Build history of the part. All positions in model axes, mm. Face numbers are marked on the shaded views. A direction names the side the tool comes from. Round coordinates to 2 decimals unless told otherwise and drop trailing zeros. Loops run counter-clockwise (first coordinate to the right, second up) from the corner with the lowest first, then second, coordinate; pieces in that order, holes last. Notation, with made-up numbers: (-30, 81.25) -> (-20, 81.25) arc R18 cw to (-20, 109.25) -> close; hole circle Ø9 at (0, 74). An arc over 180 degrees is marked (long way). Put each result on its own line as item: value. Start each with the question number.
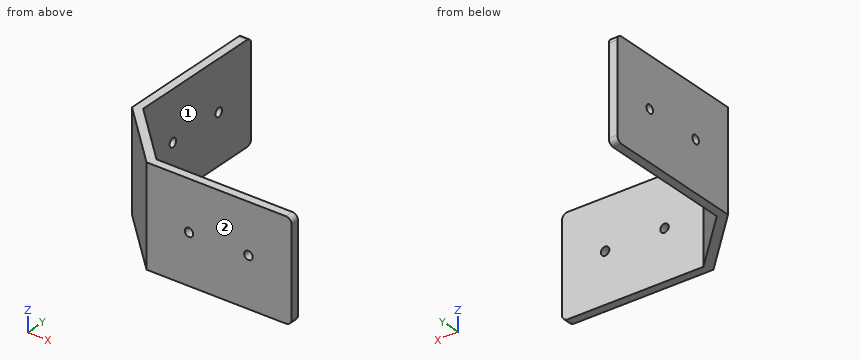
```python
from build123d import *

# Parameters (mm, degrees)
EXTRU_MINCE1_DEPTH      = 35
CONG_3_R                = 2
CONG_4_R                = 2
CONG_5_R                = 2
CONG_6_R                = 2
ESQUISSE2_R             = 1.5
ENL_V_MAT_EXTRU_1_DEPTH = 10
ESQUISSE3_R             = 1.5
ENL_V_MAT_EXTRU_2_DEPTH = 10


with BuildPart() as part:
    # Esquisse1 → Extru.-Mince1 (new body)
    with BuildSketch(Plane.XY):
        Polygon((70, -20), (20, -20), (0, 0), (0, 50), (-3, 50), (-3, -1.242640687), (18.757359313, -23), (70, -23), align=None)
    extrude(amount=EXTRU_MINCE1_DEPTH)

    # Congé3
    cong_3_edges = [part.edges().sort_by_distance(p)[0] for p in [
        (-1.5, 50, 35),
    ]]
    fillet(cong_3_edges, radius=CONG_3_R)

    # Congé4
    cong_4_edges = [part.edges().sort_by_distance(p)[0] for p in [
        (-1.5, 50, 0),
    ]]
    fillet(cong_4_edges, radius=CONG_4_R)

    # Congé5
    cong_5_edges = [part.edges().sort_by_distance(p)[0] for p in [
        (70, -21.5, 35),
    ]]
    fillet(cong_5_edges, radius=CONG_5_R)

    # Congé6
    cong_6_edges = [part.edges().sort_by_distance(p)[0] for p in [
        (70, -21.5, 0),
    ]]
    fillet(cong_6_edges, radius=CONG_6_R)

    # Esquisse2 → Enlèv. mat.-Extru.1 (cut)
    with BuildSketch(Plane.XZ.offset(23)):
        with Locations(Location((33.757359313, 17.5, 0), (0, 0, 270))):
            Circle(ESQUISSE2_R)
        with Locations(Location((54.757359313, 17.5, 0), (0, 0, 270))):
            Circle(ESQUISSE2_R)
    extrude(amount=-ENL_V_MAT_EXTRU_1_DEPTH, mode=Mode.SUBTRACT)

    # Esquisse3 → Enlèv. mat.-Extru.2 (cut)
    with BuildSketch(Plane.ZY.offset(3)):
        with Locations((17.5, 35)):
            Circle(ESQUISSE3_R)
        with Locations((17.5, 13.757359313)):
            Circle(ESQUISSE3_R)
    extrude(amount=-ENL_V_MAT_EXTRU_2_DEPTH, mode=Mode.SUBTRACT)


solid = part.part
```
Item 1: Cut at A-A on z = 17.5. Write the cut outline in (x, y), then the cut area to 3 significant figures.
Item 2: Wall check: line 1 (Y direction, x = -1.6, z = 17.5); line 2 (X direction, y = -21.45, z = 17.5); line 3 (Y direction, x = -1.3, z = 17.5). Give the ranges that are in metal, low to high. Write a range as from..to.
Item 3: Drop flat-ended pins along their axis: pin 1 (12 mm diameter, centred on x = 9.5, z = 8.5, fed in from -Y); pin 2 (12 mm diameter, centred on y = 12.5, z = 25.5, fed in from +X); pin 3 (6 mm diameter, centred on y = -13, z = 20, fed in from +X). Give the stop position or say it passes through.
Item 4: Cut at B-B on y = 35. Write the cut outline in (x, z), then the cut area to 3 significant figures.
Item 5: Cut at C-C on z = 9.5. Write the cut outline in (x, y).
Item 6: 3-axis set-ups, long thin cutter, end or side, ignore diameter. For the marked faces 1 and 2: which of +Z, -Z, +X, -X, +Y, -Y reach the whole face in a straight line?
Item 7: Cut at D-D on y = 24. Write the cut outline in (x, z).
Ans:
1. outline: (-3, -1.24) -> (18.76, -23) -> (32.26, -23) -> (32.26, -20) -> (20, -20) -> (0, 0) -> (0, 12.26) -> (-3, 12.26) -> close; (-3, 15.26) -> (0, 15.26) -> (0, 33.5) -> (-3, 33.5) -> close; (-3, 36.5) -> (0, 36.5) -> (0, 50) -> (-3, 50) -> close; (35.26, -23) -> (53.26, -23) -> (53.26, -20) -> (35.26, -20) -> close; (56.26, -23) -> (70, -23) -> (70, -20) -> (56.26, -20) -> close
1. area: 356 mm2
2. line 1: y = -2.64..12.26, 15.26..33.5, 36.5..50
2. line 2: x = 17.21..32.26, 35.26..53.26, 56.26..70
2. line 3: y = -2.94..12.26, 15.26..33.5, 36.5..50
3. pin 1: stops at y = -19.74
3. pin 2: stops at x = 0
3. pin 3: stops at x = 16
4. outline: (-3, 0) -> (0, 0) -> (0, 16) -> (-3, 16) -> close; (-3, 19) -> (0, 19) -> (0, 35) -> (-3, 35) -> close
4. area: 96.0 mm2
5. outline: (-3, -1.24) -> (18.76, -23) -> (70, -23) -> (70, -20) -> (20, -20) -> (0, 0) -> (0, 50) -> (-3, 50) -> close
6. face 1: +Z, -Z, +X, +Y
6. face 2: +Z, -Z, +X, -X, -Y
7. outline: (-3, 0) -> (0, 0) -> (0, 35) -> (-3, 35) -> close
